Build history of the part. All positions in model axes, mm. Coordinates: 2 decimals unless noted, no trailing zeros. Loops run counter-clockwise (first coordinate to the right, second up) from the corner with the lowest first, then second, coordinate; pieces in that order, holes last.
Item 1: Drill centre lines: line 1 along Y through (x, z) = (-80, 0.3); line 2 along Y through (x, z) = (-61, -0.4); line 3 along X through (y, z) = (13.5, 1.35). Where is each one in solid material? Low to high.
Item 2: Cut at A-A (y = -38.75). List the corners of the cut face in (x, z).
Item 3: Cut at B-B (x = 0). List the corners of the cut face in (y, z), and give its area (4 significant figures).
Item 4: Mould opens along X. For faces 1 (the face through (-22, 0, 0)), 2 (the face through (-87.15, 65.74, -0.02)), 3 (the face through (-81.847, 39.516, 0.021)) say: released by +X, released by -X, zero draft, split by the parting line, or undercut.
Item 5: Cut at D-D (x = 40). List the corners of the cut face in (y, z), and give its area (4 significant figures).
Item 6: Cut at C-C (y = 20). List the corners of the cut face in (x, z), and give its area (3 significant figures).
from build123d import *

# Parameters (mm, degrees)
SKETCH_1_R          = 2.0000000000000013
SKETCH_1_R_2        = 2.000000000000003
SKETCH_1_R_3        = 1.9999999999999987
EXTRUDE_1_DEPTH     = 1.5
FILLET_1_R          = 10
SKETCH_3_R          = 1.9999999999999967
SKETCH_3_R_2        = 2.0000000000000036
CUT_EXTRUDE_4_DEPTH = 114.29414150784675


with BuildPart() as part:
    # 草图1 → 凸台-拉伸1 (new, symmetric)
    with BuildSketch(Plane.XY):
        Polygon((-90, -68.75000000000003), (90, -68.75), (90, 68.75), (-90, 68.74999999999997), align=None)
        with Locations((-1.22e-15, -20)):
            Circle(SKETCH_1_R, mode=Mode.SUBTRACT)
        with Locations((-20, 0)):
            Circle(SKETCH_1_R_2, mode=Mode.SUBTRACT)
        with BuildLine():
            Line((-15.909902576697288, 12.374368670764625), (-12.374368670764548, 15.909902576697364))
            Line((-12.374368670764548, 15.909902576697364), (-8.690483378709542, 12.226017284642358))
            ThreePointArc((-8.690483378709553, 12.226017284642344), (5.421e-14, 15.000000000000014), (8.690483378709638, 12.226017284642284))
            Line((8.69048337870963, 12.226017284642296), (12.374368670764623, 15.909902576697288))
            Line((12.374368670764623, 15.909902576697288), (15.909902576697364, 12.37436867076455))
            Line((15.909902576697364, 12.37436867076455), (12.226017284642353, 8.690483378709539))
            ThreePointArc((12.226017284642342, 8.690483378709551), (14.289686127932187, 4.561235618248917), (15, 1.388e-14))
            ThreePointArc((15, 1.02e-14), (14.289686127932162, -4.561235618248962), (12.226017284642253, -8.690483378709645))
            Line((12.226017284642284, -8.690483378709619), (15.909902576697288, -12.374368670764623))
            Line((15.909902576697288, -12.374368670764623), (12.37436867076455, -15.909902576697364))
            Line((12.37436867076455, -15.909902576697364), (8.690483378709526, -12.22601728464234))
            ThreePointArc((8.690483378709535, -12.226017284642328), (-5.605e-14, -14.999999999999986), (-8.690483378709638, -12.226017284642255))
            Line((-8.690483378709613, -12.226017284642284), (-12.374368670764621, -15.909902576697291))
            Line((-12.374368670764621, -15.909902576697291), (-15.90990257669736, -12.374368670764552))
            Line((-15.90990257669736, -12.374368670764552), (-12.22601728464234, -8.69048337870953))
            ThreePointArc((-12.226017284642326, -8.690483378709544), (-15, 5.568e-14), (-12.226017284642273, 8.690483378709645))
            Line((-12.226017284642293, 8.69048337870963), (-15.909902576697288, 12.374368670764625))
        make_face(mode=Mode.SUBTRACT)
        with Locations((20, 2.45e-15)):
            Circle(SKETCH_1_R_2, mode=Mode.SUBTRACT)
        with Locations((-1.22e-15, 20)):
            Circle(SKETCH_1_R_3, mode=Mode.SUBTRACT)
    extrude(amount=EXTRUDE_1_DEPTH, both=True)

    # 圆角1
    fillet_1_edges = [part.edges().sort_by_distance(p)[0] for p in [
        (-90, 68.74999999999997, 0),
        (90, 68.75, 0),
        (90, -68.75, 0),
        (-90, -68.75000000000003, 0),
    ]]
    fillet(fillet_1_edges, radius=FILLET_1_R)

    # 草图3 → 切除-拉伸4 (cut, through all)
    with BuildSketch(Plane.XY.offset(1.5)):
        with Locations((-80, -58.75000000000001)):
            Circle(SKETCH_3_R)
        with Locations((-60, -58.75000000000001)):
            Circle(SKETCH_3_R)
        with Locations((-80.00000000000001, -38.75000000000001)):
            Circle(SKETCH_3_R)
        with Locations((-39.99999999999999, -58.75000000000001)):
            Circle(SKETCH_3_R_2)
        with Locations((-80.00000000000001, -18.750000000000007)):
            Circle(SKETCH_3_R)
        with Locations(Location((80.00000000000004, -38.749999999999986, 0), (0, 0, 180))):
            Circle(SKETCH_3_R)
        with Locations(Location((60.00000000000004, -58.75, 0), (0, 0, 180))):
            Circle(SKETCH_3_R)
        with Locations(Location((80.00000000000003, -58.749999999999986, 0), (0, 0, 180))):
            Circle(SKETCH_3_R)
        with Locations((80.00000000000003, 58.749999999999986)):
            Circle(SKETCH_3_R)
        with Locations((60.00000000000004, 58.75)):
            Circle(SKETCH_3_R)
        with Locations((80.00000000000004, 38.749999999999986)):
            Circle(SKETCH_3_R)
        with Locations(Location((-80.00000000000001, 38.75000000000001, 0), (0, 0, 180))):
            Circle(SKETCH_3_R)
        with Locations(Location((-60, 58.75000000000001, 0), (0, 0, 180))):
            Circle(SKETCH_3_R)
        with Locations(Location((-80, 58.75000000000001, 0), (0, 0, 180))):
            Circle(SKETCH_3_R)
        with Locations(Location((39.99999999999999, -58.75000000000001, 0), (0, 0, 180))):
            Circle(SKETCH_3_R_2)
        with Locations(Location((80.00000000000001, -18.750000000000007, 0), (0, 0, 180))):
            Circle(SKETCH_3_R)
    extrude(amount=-CUT_EXTRUDE_4_DEPTH, mode=Mode.SUBTRACT)


solid = part.part
Filled sheet:
1. line 1: y = -68.75 to -60.75, -56.75 to -40.75, -36.75 to -20.75, -16.75 to 36.75, 40.75 to 56.75, 60.75 to 68.75
1. line 2: y = -68.75 to -60.48, -57.02 to 57.02, 60.48 to 68.75
1. line 3: x = -90 to -14.78, -9.96 to -6.54, 6.54 to 9.96, 14.78 to 90
2. outline: (-90, -1.5) - (-82, -1.5) - (-82, 1.5) - (-90, 1.5) - close; (-78, -1.5) - (78, -1.5) - (78, 1.5) - (-78, 1.5) - close; (82, -1.5) - (90, -1.5) - (90, 1.5) - (82, 1.5) - close
3. outline: (-68.75, -1.5) - (-22, -1.5) - (-22, 1.5) - (-68.75, 1.5) - close; (-18, -1.5) - (-15, -1.5) - (-15, 1.5) - (-18, 1.5) - close; (15, -1.5) - (18, -1.5) - (18, 1.5) - (15, 1.5) - close; (22, -1.5) - (68.75, -1.5) - (68.75, 1.5) - (22, 1.5) - close
3. area: 298.5 mm2
4. face 1: undercut
4. face 2: released by -X
4. face 3: undercut
5. outline: (-68.75, -1.5) - (-60.75, -1.5) - (-60.75, 1.5) - (-68.75, 1.5) - close; (-56.75, -1.5) - (68.75, -1.5) - (68.75, 1.5) - (-56.75, 1.5) - close
5. area: 400.5 mm2
6. outline: (-90, -1.5) - (-2, -1.5) - (-2, 1.5) - (-90, 1.5) - close; (2, -1.5) - (90, -1.5) - (90, 1.5) - (2, 1.5) - close
6. area: 528 mm2
